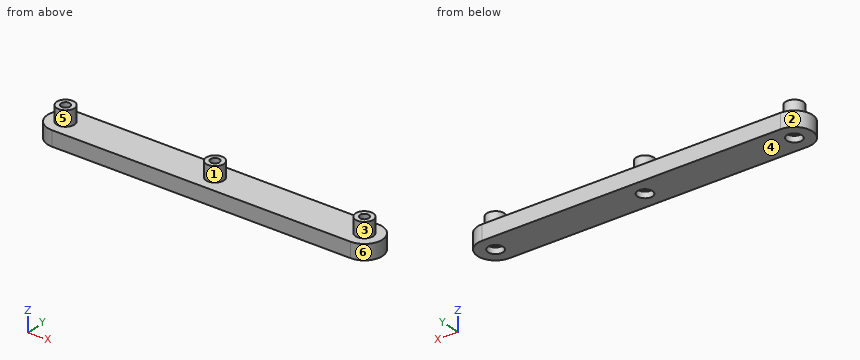
from build123d import *

# Parameters (mm, degrees)
SKETCH1_R           = 1.5
BOSS_EXTRUDE1_DEPTH = 5
SKETCH2_R           = 2.95
SKETCH2_R_2         = 1.5
BOSS_EXTRUDE2_DEPTH = 5
SKETCH4_R           = 2.5
CUT_EXTRUDE1_DEPTH  = 2


with BuildPart() as part:
    # Sketch1 → Boss-Extrude1 (new body)
    with BuildSketch(Plane.XY):
        with BuildLine():
            Line((-50, 6), (50, 6))
            ThreePointArc((50, 6), (56, 0), (50, -6))
            Line((50, -6), (-50, -6))
            ThreePointArc((-50, -6), (-56, 0), (-50, 6))
        make_face()
        with Locations((-50, 0)):
            Circle(SKETCH1_R, mode=Mode.SUBTRACT)
        with Locations((50, 0)):
            Circle(SKETCH1_R, mode=Mode.SUBTRACT)
        Circle(SKETCH1_R, mode=Mode.SUBTRACT)
    extrude(amount=BOSS_EXTRUDE1_DEPTH)

    # Sketch2 → Boss-Extrude2 (add)
    # profile 1 of 3: a face of its own
    with BuildSketch(Plane.XY.offset(5)):
        with Locations((-50, 0)):
            Circle(SKETCH2_R)
        with Locations((-50, 0)):
            Circle(SKETCH2_R_2, mode=Mode.SUBTRACT)
    # profile 2 of 3: a face of its own
    with BuildSketch(Plane.XY.offset(5)):
        Circle(SKETCH2_R)
        Circle(SKETCH2_R_2, mode=Mode.SUBTRACT)
    # profile 3 of 3: a face of its own
    with BuildSketch(Plane.XY.offset(5)):
        with Locations((50, 0)):
            Circle(SKETCH2_R)
        with Locations((50, 0)):
            Circle(SKETCH2_R_2, mode=Mode.SUBTRACT)
    extrude(amount=BOSS_EXTRUDE2_DEPTH)

    # Sketch4 → Cut-Extrude1 (cut)
    with BuildSketch(Plane(origin=(0, 0, 0), x_dir=(-1, 0, 0), z_dir=(0, 0, -1))):
        with Locations((-50, 0)):
            Circle(SKETCH4_R)
        Circle(SKETCH4_R)
        with Locations((50, 0)):
            Circle(SKETCH4_R)
    extrude(amount=-CUT_EXTRUDE1_DEPTH, mode=Mode.SUBTRACT)


solid = part.part
Read the model definition and answer for the solid it produces. Units are mm, in the model's axes. Face numbers are marked on the shaded views. A direction names the side the tool comes from. Round coordinates to 2 decimals unless told otherwise and drop trailing zeros. Loops run counter-clockwise (first coordinate to the right, second up) from the corner with the lowest first, then second, coordinate; pieces in that order, holes last.
Q1. Section D-D on y = 0 is taken. Give the number of separate pieces and of enclosed holes in the cut face, and give its area (4 significant figures).
Q2. Section B-B on x = 0 is taken. Write down the section's boundary in (y, z), and give its area (3 significant figures).
Q3. Section A-A on z = 8 is taken. Write down the section's boundary in (x, y).
Q4. Determine the mould class of the marked faces 1, 2, 3 and 4 for opening direction X: released by +X, released by -X, zero draft, split by the parting line, or undercut.
Q5. Section C-C on z = 4 is taken. Write down the section's boundary in (x, y).
Q6. Consider probe 1 along X at (y, z) = (0, 4); probe 2 along Y at (x, z) = (50, 5.25); probe 3 along X at (y, z) = (1.25, 5.5). Determine where each line is inside the solid, lowest interval first.
Q7. Each of these flat-tipped pins is pushed along its axis until it touches: pin 1 (1 mm diameter, centred on x = -36.5, y = -1.5, fed in from +Z); pin 2 (2.5 mm diameter, centred on x = 0.5, y = -0.5, fed in from -Z). Where does it stop, or does it pass through?
Q8. Which of the six approach directions +Z, -Z, +X, -X, +Y, -Y give full straight-line access (tool end or side, diameter ignored) to the marked faces 5 and 6?
Output:
1. separate pieces: 4
1. enclosed holes: 0
1. area: 546.5 mm2
2. outline: (-6, 0) - (-2.5, 0) - (-2.5, 2) - (-1.5, 2) - (-1.5, 10) - (-2.95, 10) - (-2.95, 5) - (-6, 5) - close; (1.5, 2) - (2.5, 2) - (2.5, 0) - (6, 0) - (6, 5) - (2.95, 5) - (2.95, 10) - (1.5, 10) - close
2. area: 55.5 mm2
3. outline: circle Ø5.9 at (-50, 0); circle Ø5.9 at (0, 0); circle Ø5.9 at (50, 0); hole circle Ø3 at (-50, 0); hole circle Ø3 at (0, 0); hole circle Ø3 at (50, 0)
4. face 1: undercut
4. face 2: released by -X
4. face 3: undercut
4. face 4: zero draft
5. outline: (-50, -6) - (50, -6) arc R6 ccw to (50, 6) - (-50, 6) arc R6 ccw to start; hole circle Ø3 at (-50, 0); hole circle Ø3 at (0, 0); hole circle Ø3 at (50, 0)
6. probe 1: x = -56 to -51.5, -48.5 to -1.5, 1.5 to 48.5, 51.5 to 56
6. probe 2: y = -2.95 to -1.5, 1.5 to 2.95
6. probe 3: x = -52.67 to -50.83, -49.17 to -47.33, -2.67 to -0.83, 0.83 to 2.67, 47.33 to 49.17, 50.83 to 52.67
7. pin 1: stops at z = 5
7. pin 2: stops at z = 2
8. face 5: +Z
8. face 6: +Z, -Z, +X
